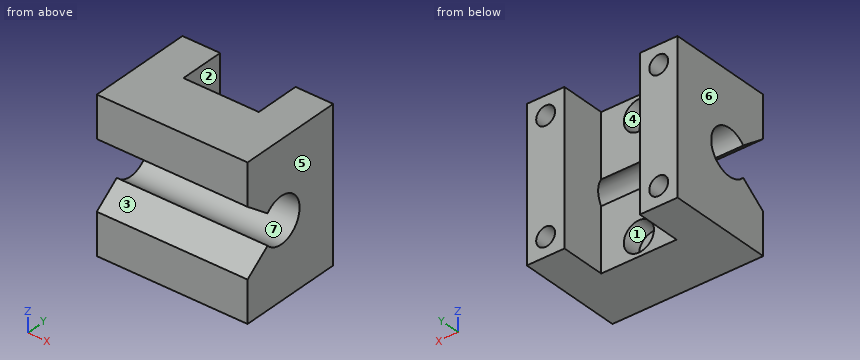
from build123d import *

# Parameters (mm, degrees)
EXTRUDE_1_DEPTH          = 20
CUT_EXTRUDE_1_DEPTH      = 32.559467676
CUT_EXTRUDE_1_DEPTH_BACK = 32.559467676
SKETCH_2_W               = 20
SKETCH_2_H               = 19.616393828
SKETCH_3_R               = 4
CUT_EXTRUDE_2_DEPTH      = 5
SKETCH_4_R               = 2.5
CUT_EXTRUDE_3_DEPTH      = 10


with BuildPart() as part:
    # Эскиз1 → Бобышка-Вытянуть1 (new, symmetric)
    with BuildSketch(Plane(origin=(0, 0, 0), x_dir=(0, 0, -1), z_dir=(1, 0, 0))):
        with BuildLine():
            Line((-4, -7.472135955), (-9, -14))
            Line((-9, -14), (-20, -14))
            Line((-20, -14), (-20, 14))
            Line((-20, 14), (20, 14))
            Line((20, 14), (20, -14))
            Line((20, -14), (9, -14))
            Line((9, -14), (4, -7.472135955))
            ThreePointArc((4, -7.472135955), (0, 3), (-4, -7.472135955))
        make_face()
    extrude(amount=EXTRUDE_1_DEPTH, both=True)

    # Эскиз2 → Вырез-Вытянуть1 (cut, two sides: drawn at the far end of the back side and taken through both)
    with BuildSketch(Plane.XY.offset(-CUT_EXTRUDE_1_DEPTH_BACK)):
        with Locations((0, 11.808196914)):
            Rectangle(SKETCH_2_W, SKETCH_2_H)
    extrude(amount=CUT_EXTRUDE_1_DEPTH + CUT_EXTRUDE_1_DEPTH_BACK, mode=Mode.SUBTRACT)

    # Эскиз3 → Вырез-Вытянуть2 (cut)
    with BuildSketch(Plane(origin=(0, 2, 0), x_dir=(1, 0, 0), z_dir=(0, 1, 0))):
        with Locations(Location((0, 15, 0), (0, 0, 270))):
            Circle(SKETCH_3_R)
        with Locations(Location((0, -15, 0), (0, 0, 270))):
            Circle(SKETCH_3_R)
    extrude(amount=-CUT_EXTRUDE_2_DEPTH, mode=Mode.SUBTRACT)

    # Эскиз4 → Вырез-Вытянуть3 (cut)
    with BuildSketch(Plane(origin=(0, 14, 0), x_dir=(1, 0, 0), z_dir=(0, 1, 0))):
        with Locations(Location((-15, 15, 0), (0, 0, 270))):
            Circle(SKETCH_4_R)
        with Locations(Location((-15, -15, 0), (0, 0, 270))):
            Circle(SKETCH_4_R)
        with Locations(Location((15, -15, 0), (0, 0, 270))):
            Circle(SKETCH_4_R)
        with Locations(Location((15, 15, 0), (0, 0, 270))):
            Circle(SKETCH_4_R)
    extrude(amount=-CUT_EXTRUDE_3_DEPTH, mode=Mode.SUBTRACT)


solid = part.part
Can you work these out from the model? Positions are in its coordinate system, mm. Face numbers are marked on the shaded views. A direction names the side the tool comes from. Coordinates: 2 decimals unless noted, no trailing zeros. Write each loop counter-clockwise with the first axis right and the second up, starting at its lowest first coordinate (ties: lowest second). Pieces come first, ordered by that corner, then holes. Notation, with made-up numbers: (-6.75, 30.25) - (43.25, 30.25) arc R34 cw to (43.25, 69.25) - close; hole circle Ø10 at (36, 43.25). An arc over 180 degrees is marked (long way). Return JSON: item names as keys, results as strings. Group by question number.
Item 1: If we section it at D-D (y = -4.25): Write out the boundary of the cut face in (x, z), then the cut area to 3 significant figures.
Item 2: I'm going to push flat-ended pins straight in: pin 1 Ø2.5 at (x, z) = (15, 16) entering from +Y; pin 2 Ø8 at (x, z) = (15, -15) entering from +Y; pin 3 Ø6.5 at (x, z) = (1.5, 14.5) entering from +Y; pin 4 Ø2.5 at (x, z) = (-1, -13.5) entering from +Y. Where does each tip first touch, or does it pass through?
Item 3: If we section it at B-B (x = 0): Write out the boundary of the cut face in (y, z).
Item 4: Please list where these lines run through material, in increasing order: probe 1 along X at (y, z) = (10.25, -15); probe 2 along X at (y, z) = (0.4, 15); probe 3 along X at (y, z) = (6, -18).
Item 5: If we section it at C-C (z = -15): Write out the boundary of the cut face in (x, y), then the cut area to 3 significant figures.
Item 6: Which directions (+Z, -Z, +X, -X, +Y, -Y) give clear straight access to the entire face, cutting with the end or side of a thin tool? Please do the marked faces 1, 2 and 3.
Item 7: If we section it at A-A (y = 8.75): Write out the boundary of the cut face in (x, z).
Item 8: We'd pull the mould along X, two halves only. Please class the marked faces 4, 5, 6 and 7: pulls with the +X half, pulls with the -X half, needs draft (parallel to the pull), parting line crosses it, or undercut.
Return value:
{
 "1": {"outline": "(-20, -20) - (20, -20) - (20, -5.87) - (-20, -5.87) - close; (-20, 5.87) - (20, 5.87) - (20, 20) - (-20, 20) - close", "area": "1,130 mm^2"},
 "2": {"pin 1": "stops at y = 4", "pin 2": "stops at y = 14", "pin 3": "stops at y = 2", "pin 4": "stops at y = -3"},
 "3": {"outline": "(-14, -20) - (2, -20) - (2, -19) - (-3, -19) - (-3, -11) - (2, -11) - (2, -3.32) arc R6 cw to (-7.47, -4) - (-14, -9) - close; (-14, 9) - (-7.47, 4) arc R6 cw to (2, 3.32) - (2, 11) - (-3, 11) - (-3, 19) - (2, 19) - (2, 20) - (-14, 20) - close"},
 "4": {"probe 1": "x = -20 to -17.5, -12.5 to -10, 10 to 12.5, 17.5 to 20", "probe 2": "x = -20 to -4, 4 to 20", "probe 3": "x = -20 to -10, 10 to 20"},
 "5": {"outline": "(-20, -14) - (20, -14) - (20, 14) - (17.5, 14) - (17.5, 4) - (12.5, 4) - (12.5, 14) - (10, 14) - (10, 2) - (4, 2) - (4, -3) - (-4, -3) - (-4, 2) - (-10, 2) - (-10, 14) - (-12.5, 14) - (-12.5, 4) - (-17.5, 4) - (-17.5, 14) - (-20, 14) - close", "area": "740 mm^2"},
 "6": {"face 1": "+Y", "face 2": "+Z, -Z, +Y", "face 3": "+X, -X, -Y"},
 "7": {"outline": "(-20, -20) - (-10, -20) - (-10, 20) - (-20, 20) - close; (10, -20) - (20, -20) - (20, 20) - (10, 20) - close; hole circle Ø5 at (-15, -15); hole circle Ø5 at (-15, 15); hole circle Ø5 at (15, -15); hole circle Ø5 at (15, 15)"},
 "8": {"face 4": "undercut", "face 5": "pulls with the +X half", "face 6": "pulls with the -X half", "face 7": "needs draft"}
}
